Read the model definition and answer for the solid it produces. Units are mm, in the model's axes. A direction names the side the tool comes from. Give positions to 0.01 mm unless a question says otherwise; leave off trailing zeros. Order: outer loops, then holes, each group sorted by start corner. A loop starts at its lowest first (then second) coordinate and runs counter-clockwise, first axis right, second up. Notation, with made-up numbers: (22, 66.25) - (26, 66.25) arc R22 cw to (26, 77.25) - close; hole circle Ø4 at (-19.75, 12). An arc over 180 degrees is marked (long way). Write each question's results on one line, items separated by ' | '.
from build123d import *

# Parameters (mm, degrees)
SKETCH1_R               = 6.985
BOSS_EXTRUDE1_DEPTH     = 6.35
SKETCH3_R               = 4.7625
CUT_EXTRUDE1_DEPTH      = 63.5
SKETCH5_W               = 76.2
SKETCH5_H               = 13.97
BOSS_EXTRUDE2_DEPTH     = 101.6
SKETCH6_W               = 50.8
SKETCH6_H               = 95.25
CUT_EXTRUDE2_DEPTH      = 116.325510621
SKETCH7_R               = 4.7625
CUT_EXTRUDE3_DEPTH      = 115.689156964
CUT_EXTRUDE4_DEPTH      = 126.436209784
CUT_EXTRUDE4_DEPTH_BACK = 19.05
SKETCH8_R               = 4.7625
CUT_EXTRUDE5_START      = -13.97
SKETCH9_R               = 1.016
CUT_EXTRUDE5_DEPTH      = 13.97


with BuildPart() as part:
    # Sketch1 → Boss-Extrude1 (new body)
    with BuildSketch(Plane(origin=(0, 0, 0), x_dir=(1, 0, 0), z_dir=(0, 1, 0))):
        with Locations(Location((0, 0, 0), (0, 0, 270))):
            Circle(SKETCH1_R)
    extrude(amount=-BOSS_EXTRUDE1_DEPTH)

    # Sketch3 → Cut-Extrude1 (cut)
    with BuildSketch(Plane(origin=(0, 0, 0), x_dir=(1, 0, 0), z_dir=(0, 1, 0))):
        with Locations(Location((0, 0, 0), (0, 0, 270))):
            Circle(SKETCH3_R)
    extrude(amount=-CUT_EXTRUDE1_DEPTH, mode=Mode.SUBTRACT)

    # Sketch5 → Boss-Extrude2 (add)
    with BuildSketch(Plane(origin=(0, -6.35, 0), x_dir=(-1, 0, 0), z_dir=(0, -1, 0))):
        Rectangle(SKETCH5_W, SKETCH5_H)
    extrude(amount=BOSS_EXTRUDE2_DEPTH)

    # Sketch6 → Cut-Extrude2 (cut, through all)
    with BuildSketch(Plane(origin=(0, 0, -6.985), x_dir=(-1, 0, 0), z_dir=(0, 0, -1))):
        with Locations((0, -60.325)):
            Rectangle(SKETCH6_W, SKETCH6_H)
    extrude(amount=-CUT_EXTRUDE2_DEPTH, mode=Mode.SUBTRACT)

    # Sketch7 → Cut-Extrude3 (cut, through all)
    with BuildSketch(Plane(origin=(0, 0, 0), x_dir=(1, 0, 0), z_dir=(0, 1, 0))):
        with Locations(Location((0, 0, 0), (0, 0, 270))):
            Circle(SKETCH7_R)
    extrude(amount=-CUT_EXTRUDE3_DEPTH, mode=Mode.SUBTRACT)

    # Sketch8 → Cut-Extrude4 (cut, two sides: drawn at the far end of the back side and taken through both)
    with BuildSketch(Plane.ZY.offset(-25.4).offset(-CUT_EXTRUDE4_DEPTH_BACK)):
        with Locations((0, -79.375)):
            Circle(SKETCH8_R)
    extrude(amount=CUT_EXTRUDE4_DEPTH + CUT_EXTRUDE4_DEPTH_BACK, mode=Mode.SUBTRACT)

    # Sketch9 → Cut-Extrude5 (cut)
    with BuildSketch(Plane.XY.offset(6.985).offset(CUT_EXTRUDE5_START)):
        with Locations(Location((0, -6.35, 0), (0, 0, 90))):
            Circle(SKETCH9_R)
    extrude(amount=CUT_EXTRUDE5_DEPTH, mode=Mode.SUBTRACT)


solid = part.part
(1) Section C-C (x = 10.5) is taken. Give the vertices of the cut face in (y, z) (3 decimals).
Conclusion:
outline: (-12.7, -6.985) - (-6.35, -6.985) - (-6.35, 6.985) - (-12.7, 6.985) - close
(2) Section A-A (z = 0) is taken. State how many separate pieces and enclosed holes the cut face has, plus the area to 3 significant figures.
Conclusion:
separate pieces: 4 | enclosed holes: 0 | area: 2,630 mm^2
(3) The mould has two halves that part along Z. Classify faces 3 (the face through (20, -6.35, 0)), 4 (the face through (-31.661, -74.653, -0.62)), 5 (the face through (2.1, -3.13, 6.66)): pulls with the +Z half, pulls with the -Z half, needs draft (parallel to the pull), parting line crosses it, or undercut.
Conclusion:
face 3: needs draft | face 4: undercut | face 5: parting line crosses it
(4) This flat-tipped pin is pushed along its axis until it touches: pin 1 (4 mm diameter, centred on x = -11.5, z = 1.5, fed in from +Y). Where does it stop, or does it pass through?
Conclusion:
pin 1: y = -6.35
(5) Section B-B (y = -86.5) is taken. Give the vertices of the cut face in (x, z) (3 decimals), plus the area to 3 significant figures.
Conclusion:
outline: (-38.1, -6.985) - (-25.4, -6.985) - (-25.4, 6.985) - (-38.1, 6.985) - close; (25.4, -6.985) - (38.1, -6.985) - (38.1, 6.985) - (25.4, 6.985) - close | area: 355 mm^2
(6) For faces 1 (the face through (38.1, -56, 0)), 2 (the face through (0, -12.7, -5)), determine the directions among +Z, -Z, +X, -X, +Y, -Y from which every point of the face is accessible in a straight line to the end or side of a thin tool.
Conclusion:
face 1: +Z, -Z, +X, +Y, -Y | face 2: +Z, -Z, -Y
(7) Consider probe 1 along X at (y, z) = (-58.5, 5.25); probe 2 along Y at (x, z) = (0, 5.65); probe 3 along Y at (x, z) = (-14.5, 4.5). Determine where each line is inside the solid, lowest interval first. Write a range as [from, to].
Conclusion:
probe 1: [-38.1, -25.4], [25.4, 38.1] | probe 2: [-12.7, -7.37], [-5.33, 0] | probe 3: [-12.7, -6.35]
